Autodesk Inventor part; units mm, degrees
ref_plane "YZ Plane" through (0, 0, 0) normal (1, 0, 0) x (0, 1, 0)
ref_plane "XZ Plane" through (0, 0, 0) normal (0, 1, 0) x (-1, 0, 0)
ref_plane "XY Plane" through (0, 0, 0) normal (0, 0, 1) x (1, 0, 0)
sketch "Sketch1" plane through (0, 0, 0) normal (0, 0, 1) x (1, 0, 0)
  circle A0 centre (-17.78, 18.415) radius 1.7525
  circle A1 centre (17.7801, 18.4151) radius 1.7525
  circle A2 centre (-17.78, -18.4151) radius 1.7525
  circle A3 centre (17.7799, -18.415) radius 1.7525
  line L0 (6.35, -18.415) -> (-6.35, -18.415)
  line L1 (-6.35, -18.415) -> (-6.35, -22.5171)
  line L2 (-6.35, -22.5171) -> (-27.94, -22.5171)
  line L3 (-27.94, -22.5171) -> (-27.94, 22.513)
  line L4 (-27.94, 22.513) -> (27.94, 22.513)
  line L5 (27.94, 22.513) -> (27.94, -22.5171)
  line L6 (27.94, -22.5171) -> (6.35, -22.5171)
  line L7 (6.35, -22.5171) -> (6.35, -18.415)
  line L8 (16.0276, 15.875) -> (25.4, 15.875)
  line L9 (25.4, 15.875) -> (25.4, -15.875)
  line L10 (25.4, -15.875) -> (-25.4, -15.875)
  line L11 (-25.4, -15.875) -> (-25.4, 15.875)
  line L12 (-25.4, 15.875) -> (-16.0274, 15.875)
  line L13 (-16.0274, 15.875) -> (-13.4874, 19.194)
  line L14 (-13.4874, 19.194) -> (13.4876, 19.194)
  line L15 (13.4876, 19.194) -> (16.0276, 15.875)
  point P0 (0, 0)
extrude "Extrusion1" add sketch "Sketch1" along normal blind 2.8956
properties part number "battery_mount"
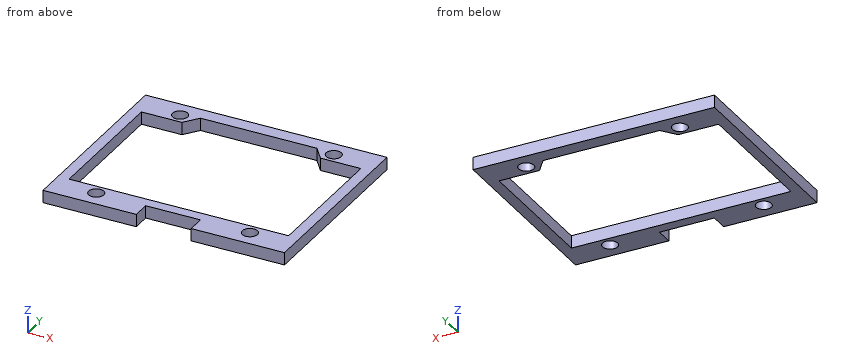
The model under review builds one solid part; all positions refer to its coordinate system, in mm. Coordinates: 2 decimals unless noted, no trailing zeros. Write each loop counter-clockwise with the first axis right and the second up, starting at its lowest first coordinate (ties: lowest second). Pieces come first, ordered by that corner, then holes. Notation, with made-up numbers: (66, -8.5) - (75, -8.5) arc R29 cw to (75, 11.5) - close; hole circle Ø4 at (67.25, 1.25). An arc over 180 degrees is marked (long way). Write item = value, one per line.
(1) Consider section D-D, the plane z = 2.45. State how many separate pieces and enclosed holes the cut face has, then the cut area to 3 significant figures.
Result sheet:
separate_pieces = 1
enclosed_holes = 5
area = 715 mm^2
(2) Consider section A-A, the plane x = 24. Give the boundary of the cut face in (y, z) (3 decimals).
Result sheet:
outline = (-22.517, 0) - (-15.875, 0) - (-15.875, 2.896) - (-22.517, 2.896) - close; (15.875, 0) - (22.513, 0) - (22.513, 2.896) - (15.875, 2.896) - close
(3) Consider section C-C, the plane x = -17.78. Give the boundary of the cut face in (y, z) (1 decimal).
Result sheet:
outline = (-22.5, 0) - (-20.2, 0) - (-20.2, 2.9) - (-22.5, 2.9) - close; (-16.7, 0) - (-15.9, 0) - (-15.9, 2.9) - (-16.7, 2.9) - close; (15.9, 0) - (16.7, 0) - (16.7, 2.9) - (15.9, 2.9) - close; (20.2, 0) - (22.5, 0) - (22.5, 2.9) - (20.2, 2.9) - close
(4) For line 1 (Y direction, x = -17.78, z = 2.1) (1 decimal); line 2 (X direction, y = -15.5, z = 0.6); line 3 (Y direction, x = -5.5, z = 0.3) (3 decimals), list the stretches that pass through material, from the lowest coordinate up. Write a range as [from, to].
Result sheet:
line_1 = [-22.5, -20.2], [-16.7, -15.9], [15.9, 16.7], [20.2, 22.5]
line_2 = [-27.94, -25.4], [25.4, 27.94]
line_3 = [-18.415, -15.875], [19.194, 22.513]
(5) Consider section B-B, the plane y = -5. Give the boundary of the cut face in (x, z), then the cut area to 3 significant figures.
Result sheet:
outline = (-27.94, 0) - (-25.4, 0) - (-25.4, 2.9) - (-27.94, 2.9) - close; (25.4, 0) - (27.94, 0) - (27.94, 2.9) - (25.4, 2.9) - close
area = 14.7 mm^2
